Here's how the part is built. I have some questions about the finished solid (model axes, mm). A direction names the side the tool comes from. Round coordinates to 2 decimals unless told otherwise and drop trailing zeros. Loops run counter-clockwise (first coordinate to the right, second up) from the corner with the lowest first, then second, coordinate; pieces in that order, holes last. Notation, with made-up numbers: M -14.5,10 L -3.5,10 A26 ccw -3.5,47 Z; hole C 80,67 d6. An arc over 180 degrees is marked long. One line per question, with ' | ' between items. Start each with the question number.
Autodesk Inventor part; units mm, degrees
ref_plane "YZ Plane" through (0, 0, 0) normal (1, 0, 0) x (0, 1, 0)
ref_plane "XZ Plane" through (0, 0, 0) normal (0, 1, 0) x (-1, 0, 0)
ref_plane "XY Plane" through (0, 0, 0) normal (0, 0, 1) x (1, 0, 0)
sketch "Sketch1" plane through (0, 0, 0) normal (0, 0, 1) x (1, 0, 0)
  line L0 (-1.5495, 0.6331) -> (-0.724, 3.4271)
  line L1 (-0.724, 3.4271) -> (0.1015, 0.6331)
  line L2 (0.1015, 0.6331) -> (-1.5495, 0.6331) construction
  line L3 (-0.724, 0.6331) -> (-0.724, 0.8628) construction
  line L4 (-3.0816, -0.0934) -> (-3.5501, 2.7821)
  line L5 (-3.5501, 2.7821) -> (-1.5941, 0.623)
  line L6 (-4.1468, -1.4127) -> (-5.8165, 0.9748)
  line L7 (-5.8165, 0.9748) -> (-3.1174, -0.1219)
  line L8 (-4.534, -3.0635) -> (-7.0742, -1.637)
  line L9 (-7.0742, -1.637) -> (-4.1666, -1.4539)
  line L10 (-4.1666, -4.7188) -> (-7.0742, -4.5357)
  line L11 (-7.0742, -4.5357) -> (-4.534, -3.1092)
  line L12 (-3.1174, -6.0508) -> (-5.8165, -7.1474)
  line L13 (-5.8165, -7.1474) -> (-4.1468, -4.76)
  line L14 (-1.5941, -6.7957) -> (-3.5501, -8.9548)
  line L15 (-3.5501, -8.9548) -> (-3.0816, -6.0793)
  line L16 (0.1015, -6.8058) -> (-0.724, -9.5998)
  line L17 (-0.724, -9.5998) -> (-1.5495, -6.8058)
  line L18 (1.6335, -6.0793) -> (2.1021, -8.9548)
  line L19 (2.1021, -8.9548) -> (0.146, -6.7957)
  line L20 (2.6987, -4.76) -> (4.3684, -7.1474)
  line L21 (4.3684, -7.1474) -> (1.6693, -6.0508)
  line L22 (3.0859, -3.1092) -> (5.6261, -4.5357)
  line L23 (5.6261, -4.5357) -> (2.7185, -4.7188)
  line L24 (2.7185, -1.4539) -> (5.6261, -1.637)
  line L25 (5.6261, -1.637) -> (3.0859, -3.0635)
  line L26 (1.6693, -0.1219) -> (4.3684, 0.9748)
  line L27 (4.3684, 0.9748) -> (2.6987, -1.4127)
  line L28 (0.146, 0.623) -> (2.1021, 2.7821)
  line L29 (2.1021, 2.7821) -> (1.6335, -0.0934)
  arc A0 (-1.5495, 0.6331) -> (-1.5941, 0.623) centre (-0.724, -3.0863) ccw
  arc A1 (-3.0816, -0.0934) -> (-3.1174, -0.1219) centre (-0.724, -3.0863) ccw
  arc A2 (-4.1468, -1.4127) -> (-4.1666, -1.4539) centre (-0.724, -3.0863) ccw
  arc A3 (-4.534, -3.0635) -> (-4.534, -3.1092) centre (-0.724, -3.0863) ccw
  arc A4 (-4.1666, -4.7188) -> (-4.1468, -4.76) centre (-0.724, -3.0863) ccw
  arc A5 (-3.1174, -6.0508) -> (-3.0816, -6.0793) centre (-0.724, -3.0863) ccw
  arc A6 (-1.5941, -6.7957) -> (-1.5495, -6.8058) centre (-0.724, -3.0863) ccw
  arc A7 (0.1015, -6.8058) -> (0.146, -6.7957) centre (-0.724, -3.0863) ccw
  arc A8 (1.6335, -6.0793) -> (1.6693, -6.0508) centre (-0.724, -3.0863) ccw
  arc A9 (2.6987, -4.76) -> (2.7185, -4.7188) centre (-0.724, -3.0863) ccw
  arc A10 (3.0859, -3.1092) -> (3.0859, -3.0635) centre (-0.724, -3.0863) ccw
  arc A11 (2.7185, -1.4539) -> (2.6987, -1.4127) centre (-0.724, -3.0863) ccw
  arc A12 (1.6693, -0.1219) -> (1.6335, -0.0934) centre (-0.724, -3.0863) ccw
  arc A13 (0.146, 0.623) -> (0.1015, 0.6331) centre (-0.724, -3.0863) ccw
  point P0 (0, 0)
  dimension "d0" = 1.651
  dimension "d1" = 2.794
extrude "Extrusion1" add sketch "Sketch1" along normal blind 2.54
properties part number "Small Gear Phone Case Mech"
1) I'm going to push flat-ended pins straight in: pin 1 Ø1.5 at (x, z) = (4, 2) entering from +Y; pin 2 Ø1 at (x, z) = (3.5, 0.5) entering from +Y; pin 3 Ø6 at (x, y) = (-3.5, -7.5) entering from -Z. Where does each tip first touch, or does it pass through?
2) Imagine slicing it at A-A (y = -8.5). Write out the boundary of the cut face in (x, z), then the cut area to 3 significant figures.
3) For faces 4 (the face through (1.865, -7.497, 1.252)), 5 (the face through (-4.993, -5.97, 1.252)), 6 (the face through (-1.13, -8.22, 1.25)), which set-ups out of +Z, -Z, +X, -X, +Y, -Y let a thin tool reach every point of the face, with its end or its side?
4) We'd pull the mould along X, two halves only. Please class faces 1 (the face through (-2.56, -7.86, 1.25)), 2 (the face through (3.522, -5.937, 1.252)), 3 (the face through (-1, -3, 2.54)): pulls with the +X half, pulls with the -X half, needs draft (parallel to the pull), parting line crosses it, or undercut.
5) Please list where these lines run through material, in increasing order: L1, parallel to Y at x = 4, z = 1.65; L2, parallel to Y at x = -5.25, z = 1.8; L3, parallel to X at y = 0.25, z = 1.25. Write a range as from..to.
6) Imagine slicing it at C-C (y = -7). Write out the boundary of the cut face in (x, z).
7) Imagine slicing it at D-D (y = 1.25). Write out the boundary of the cut face in (x, z), then the cut area to 3 significant figures.
8) Imagine slicing it at B-B (x = 3.5). Write out the boundary of the cut face in (y, z).
Results are:
1) pin 1: y = 0.97 | pin 2: y = 0.83 | pin 3: z = 0
2) outline: M -3.48,0 L -3.14,0 L -3.14,2.54 L -3.48,2.54 Z; M -1.05,0 L -0.4,0 L -0.4,2.54 L -1.05,2.54 Z; M 1.69,0 L 2.03,0 L 2.03,2.54 L 1.69,2.54 Z | area: 3.37 mm²
3) face 4: +Z, -Z | face 5: +Z, -Z, -X | face 6: +Z, -Z, -Y
4) face 1: undercut | face 2: pulls with the +X half | face 3: needs draft
5) L1: -7..-6.62, -4.64..-3.62, -2.55..-1.53, 0.45..0.83 | L2: -6.92..-6.34, -4.65..-3.51, -2.66..-1.52, 0.16..0.74 | L3: -5.31..-4.03, -3.14..1.69, 2.58..3.86
6) outline: M -5.71,0 L -5.45,0 L -5.45,2.54 L -5.71,2.54 Z; M -3.23,0 L -1.78,0 L -1.78,2.54 L -3.23,2.54 Z; M -1.49,0 L 0.04,0 L 0.04,2.54 L -1.49,2.54 Z; M 0.33,0 L 1.78,0 L 1.78,2.54 L 0.33,2.54 Z; M 4.01,0 L 4.27,0 L 4.27,2.54 L 4.01,2.54 Z
7) outline: M -3.3,0 L -2.16,0 L -2.16,2.54 L -3.3,2.54 Z; M -1.37,0 L -0.08,0 L -0.08,2.54 L -1.37,2.54 Z; M 0.71,0 L 1.85,0 L 1.85,2.54 L 0.71,2.54 Z | area: 9.05 mm²
8) outline: M -6.79,0 L -5.91,0 L -5.91,2.54 L -6.79,2.54 Z; M -4.67,0 L -3.34,0 L -3.34,2.54 L -4.67,2.54 Z; M -2.83,0 L -1.5,0 L -1.5,2.54 L -2.83,2.54 Z; M -0.27,0 L 0.62,0 L 0.62,2.54 L -0.27,2.54 Z
